```python
from build123d import *

# Parameters (mm, degrees)
SKETCH1_W                    = 510.0574
SKETCH1_H                    = 446.1002
BOSS_EXTRUDE1_DEPTH          = 0.9144
SKETCH6_W                    = 177.8
SKETCH6_H                    = 177.8
CUT_EXTRUDE1_DEPTH           = 0.9144
EDGE_FLANGE1_STRIP_W         = 5.4864
EDGE_FLANGE1_STRIP_H         = 0.9144
EDGE_FLANGE1_STRIP_CUT_DEPTH = 446.1002
EDGE_FLANGE1_DEPTH           = 446.1002
EDGE_FLANGE2_STRIP_W         = 5.4864
EDGE_FLANGE2_STRIP_H         = 0.9144
EDGE_FLANGE2_STRIP_CUT_DEPTH = 446.1002
EDGE_FLANGE2_DEPTH           = 446.1002
SKETCH13_R                   = 3.2639
CUT_EXTRUDE2_DEPTH           = 2.54
SKETCH17_R                   = 3.175
CUT_EXTRUDE5_DEPTH           = 12.7
SKETCH18_R                   = 3.2639
CUT_EXTRUDE6_DEPTH           = 12.7
SKETCH19_R                   = 3.2639
CUT_EXTRUDE7_DEPTH           = 559.94900381


# Sheet-metal steps are written as plain solids
with BuildPart() as part:
    # Sketch1 → Boss-Extrude1 (new body)
    with BuildSketch(Plane(origin=(0, 0, 0), x_dir=(1, 0, 0), z_dir=(0, 1, 0))):
        Rectangle(SKETCH1_W, SKETCH1_H)
    extrude(amount=BOSS_EXTRUDE1_DEPTH)

    # Sketch6 → Cut-Extrude1 (cut)
    with BuildSketch(Plane(origin=(0, 0.9144, 0), x_dir=(1, 0, 0), z_dir=(0, 1, 0))):
        Rectangle(SKETCH6_W, SKETCH6_H)
    extrude(amount=-CUT_EXTRUDE1_DEPTH, mode=Mode.SUBTRACT)

    # Edge-Flange1 strip (across the edge) → Edge-Flange1 strip cut (cut)
    with BuildSketch(Plane(origin=(255.0287, 0.9144, 223.0501), x_dir=(-1, 0, 0), z_dir=(0, 0, -1))):
        with Locations((-1.8288, -0.4572)):
            Rectangle(EDGE_FLANGE1_STRIP_W, EDGE_FLANGE1_STRIP_H)
    extrude(amount=EDGE_FLANGE1_STRIP_CUT_DEPTH, mode=Mode.SUBTRACT)

    # Edge-Flange1 section (across the edge) → Edge-Flange1 (add)
    with BuildSketch(Plane(origin=(255.0287, 0.9144, 223.0501), x_dir=(-1, 0, 0), z_dir=(0, 0, -1))):
        with BuildLine():
            Line((-0.9144, 0.9144), (-0.9144, 24.4856))
            Line((-0.9144, 24.4856), (0, 24.4856))
            Line((0, 24.4856), (0, 0.9144))
            ThreePointArc((0, 0.9144), (0.267821559, 0.267821559), (0.9144, 0))
            Line((0.9144, 0), (0.9144, -0.9144))
            ThreePointArc((0.9144, -0.9144), (-0.378756881, -0.378756881), (-0.9144, 0.9144))
        make_face()
    extrude(amount=EDGE_FLANGE1_DEPTH)

    # Edge-Flange2 strip (across the edge) → Edge-Flange2 strip cut (cut)
    with BuildSketch(Plane(origin=(-255.0287, 0.9144, -223.0501), x_dir=(1, 0, 0), z_dir=(0, 0, 1))):
        with Locations((-1.8288, -0.4572)):
            Rectangle(EDGE_FLANGE2_STRIP_W, EDGE_FLANGE2_STRIP_H)
    extrude(amount=EDGE_FLANGE2_STRIP_CUT_DEPTH, mode=Mode.SUBTRACT)

    # Edge-Flange2 section (across the edge) → Edge-Flange2 (add)
    with BuildSketch(Plane(origin=(-255.0287, 0.9144, -223.0501), x_dir=(1, 0, 0), z_dir=(0, 0, 1))):
        with BuildLine():
            Line((-0.9144, 0.9144), (-0.9144, 24.4856))
            Line((-0.9144, 24.4856), (0, 24.4856))
            Line((0, 24.4856), (0, 0.9144))
            ThreePointArc((0, 0.9144), (0.267821559, 0.267821559), (0.9144, 0))
            Line((0.9144, 0), (0.9144, -0.9144))
            ThreePointArc((0.9144, -0.9144), (-0.378756881, -0.378756881), (-0.9144, 0.9144))
        make_face()
    extrude(amount=EDGE_FLANGE2_DEPTH)

    # Sketch13 → Cut-Extrude2 (cut)
    with BuildSketch(Plane(origin=(0, 0, 0), x_dir=(-1, 0, 0), z_dir=(0, -1, 0))):
        with Locations(Location((241.6429, 208.5213, 0), (0, 0, 90))):
            Circle(SKETCH13_R)
        with Locations(Location((241.6429, 119.6213, 0), (0, 0, 90))):
            Circle(SKETCH13_R)
        with Locations(Location((241.6429, 30.7213, 0), (0, 0, 90))):
            Circle(SKETCH13_R)
        with Locations(Location((241.6429, -58.1787, 0), (0, 0, 90))):
            Circle(SKETCH13_R)
        with Locations(Location((241.6429, -147.0787, 0), (0, 0, 90))):
            Circle(SKETCH13_R)
        with Locations(Location((-240.9571, -147.0787, 0), (0, 0, 90))):
            Circle(SKETCH13_R)
        with Locations(Location((-240.9571, -58.1787, 0), (0, 0, 90))):
            Circle(SKETCH13_R)
        with Locations(Location((-240.9571, 30.7213, 0), (0, 0, 90))):
            Circle(SKETCH13_R)
        with Locations(Location((-240.9571, 119.6213, 0), (0, 0, 90))):
            Circle(SKETCH13_R)
        with Locations(Location((-240.9571, 208.5213, 0), (0, 0, 90))):
            Circle(SKETCH13_R)
    extrude(amount=-CUT_EXTRUDE2_DEPTH, mode=Mode.SUBTRACT)

    # Sketch17 → Cut-Extrude5 (cut)
    with BuildSketch(Plane.XZ.offset(4.7498)):
        with Locations(Location((-184.4929, 169.2148, 0), (0, 0, 270))):
            Circle(SKETCH17_R)
        with Locations(Location((183.8071, 169.2148, 0), (0, 0, 270))):
            Circle(SKETCH17_R)
        with Locations(Location((183.8071, -199.0852, 0), (0, 0, 270))):
            Circle(SKETCH17_R)
        with Locations(Location((-184.4929, -199.0852, 0), (0, 0, 270))):
            Circle(SKETCH17_R)
    extrude(amount=-CUT_EXTRUDE5_DEPTH, mode=Mode.SUBTRACT)

    # Sketch18 → Cut-Extrude6 (cut)
    with BuildSketch(Plane(origin=(0, 0.9144, 0), x_dir=(1, 0, 0), z_dir=(0, 1, 0))):
        with Locations(Location((-203.5429, -188.2648, 0), (0, 0, 270))):
            Circle(SKETCH18_R)
        with Locations(Location((202.8571, 218.1352, 0), (0, 0, 270))):
            Circle(SKETCH18_R)
        with Locations(Location((-101.9429, -188.2648, 0), (0, 0, 270))):
            Circle(SKETCH18_R)
        with Locations(Location((-0.3429, -188.2648, 0), (0, 0, 270))):
            Circle(SKETCH18_R)
        with Locations(Location((101.2571, -188.2648, 0), (0, 0, 270))):
            Circle(SKETCH18_R)
        with Locations(Location((202.8571, -188.2648, 0), (0, 0, 270))):
            Circle(SKETCH18_R)
        with Locations(Location((-203.5429, -86.6648, 0), (0, 0, 270))):
            Circle(SKETCH18_R)
        with Locations(Location((-203.5429, 14.9352, 0), (0, 0, 270))):
            Circle(SKETCH18_R)
        with Locations(Location((-203.5429, 116.5352, 0), (0, 0, 270))):
            Circle(SKETCH18_R)
        with Locations((-203.5429, -289.8648)):
            Circle(SKETCH18_R)
        with Locations(Location((202.8571, 116.5352, 0), (0, 0, 270))):
            Circle(SKETCH18_R)
        with Locations((-203.5429, -391.4648)):
            Circle(SKETCH18_R)
        with Locations(Location((202.8571, 14.9352, 0), (0, 0, 270))):
            Circle(SKETCH18_R)
        with Locations((-203.5429, -493.0648)):
            Circle(SKETCH18_R)
        with Locations(Location((202.8571, -86.6648, 0), (0, 0, 270))):
            Circle(SKETCH18_R)
        with Locations((-305.1429, -188.2648)):
            Circle(SKETCH18_R)
        with Locations(Location((101.2571, 218.1352, 0), (0, 0, 270))):
            Circle(SKETCH18_R)
        with Locations((-406.7429, -188.2648)):
            Circle(SKETCH18_R)
        with Locations(Location((-0.3429, 218.1352, 0), (0, 0, 270))):
            Circle(SKETCH18_R)
        with Locations((-508.3429, -188.2648)):
            Circle(SKETCH18_R)
        with Locations(Location((-101.9429, 218.1352, 0), (0, 0, 270))):
            Circle(SKETCH18_R)
        with Locations((-609.9429, -188.2648)):
            Circle(SKETCH18_R)
        with Locations(Location((-203.5429, 218.1352, 0), (0, 0, 270))):
            Circle(SKETCH18_R)
    extrude(amount=-CUT_EXTRUDE6_DEPTH, mode=Mode.SUBTRACT)

    # Sketch19 → Cut-Extrude7 (cut, through all)
    with BuildSketch(Plane(origin=(255.9431, 0, 0), x_dir=(0, 0, -1), z_dir=(1, 0, 0))):
        with Locations(Location((-197.6501, 12.7, 0), (0, 0, 90))):
            Circle(SKETCH19_R)
        with Locations(Location((-96.0501, 12.7, 0), (0, 0, 90))):
            Circle(SKETCH19_R)
        with Locations(Location((5.5499, 12.7, 0), (0, 0, 90))):
            Circle(SKETCH19_R)
        with Locations(Location((107.1499, 12.7, 0), (0, 0, 90))):
            Circle(SKETCH19_R)
        with Locations(Location((208.7499, 12.7, 0), (0, 0, 90))):
            Circle(SKETCH19_R)
    extrude(amount=-CUT_EXTRUDE7_DEPTH, mode=Mode.SUBTRACT)


solid = part.part
```
Check sheet for the modelled part. Datum: model origin and axes. Units: mm. A direction names the side the tool comes from. Give positions to 0.01 mm unless a question says otherwise; leave off trailing zeros. Order: outer loops, then holes, each group sorted by start corner. A loop starts at its lowest first (then second) coordinate and runs counter-clockwise, first axis right, second up. Notation, with made-up numbers: (50.25, 13) -> (64.25, 13) arc R5 cw to (64.25, 19) -> close; hole circle Ø10 at (-11, -12.5). An arc over 180 degrees is marked (long way). Use CSV: the item, a comma, the result in double quotes. Start each with the question number.
1) Sectioned sample at B-B, the plane x = 38.5. Record the boundary of the cut face in (y, z).
2) Sectioned sample at C-C, the plane x = 194. Record the boundary of the cut face in (y, z).
3) Mould release check, pull along X, two halves, no side actions. Record for faces 3 (the face through (1.2, 0.5, -223.05)), 4 (the face through (255.943, 13, 3)), 5 (the face through (-255.029, 16, -3)): released by +X, released by -X, zero draft, split by the parting line, or undercut.
4) Material ranges on line 1 (X direction, y = 9.25, z = 180); line 2 (Y direction, x = 29, z = -144.5), recorded low to high. Write a range as from..to.
5) Set-up check for faces 1 (the face through (-255.943, 16, -3)), 2 (the face through (-4, 0.914, 96)): record each of +Z, -Z, +X, -X, +Y, -Y from which the full face is reachable in a straight line by a thin tool's end or side.
6) Sectioned sample at A-A, the plane y = 21.25. Record the boundary of the cut face in (x, z), plus the area to 3 significant figures.
7) Go/stop test with flat-tipped pins: P1, Ø8, axis at x = 31.5, z = 111, coming from the +Y side; P2, Ø0.7, axis at y = 0.5, z = 6.5, coming from the -X side. Record where each tip stops, or that it passes through.
Recorded:
1,outline,"(0, -223.05) -> (0.91, -223.05) -> (0.91, -88.9) -> (0, -88.9) -> close; (0, 88.9) -> (0.91, 88.9) -> (0.91, 223.05) -> (0, 223.05) -> close"
2,outline,"(0, -223.05) -> (0.91, -223.05) -> (0.91, 223.05) -> (0, 223.05) -> close"
3,face 3,"zero draft"
3,face 4,"released by +X"
3,face 5,"undercut"
4,line 1,"-255.94..-255.03, 255.03..255.94"
4,line 2,"0..0.91"
5,face 1,"+Z, -Z, -X, +Y, -Y"
5,face 2,"+Z, -Z, +Y"
6,outline,"(-255.94, -223.05) -> (-255.03, -223.05) -> (-255.03, 223.05) -> (-255.94, 223.05) -> close; (255.03, -223.05) -> (255.94, -223.05) -> (255.94, 223.05) -> (255.03, 223.05) -> close"
6,area,"816 mm2"
7,P1,"y = 0.91"
7,P2,"x = -255.66"
